Build history of the part. All positions in model axes, mm. Give positions to 0.01 mm unless a question says otherwise; leave off trailing zeros. Write each loop counter-clockwise with the first axis right and the second up, starting at its lowest first coordinate (ties: lowest second). Pieces come first, ordered by that corner, then holes.
from build123d import *

# Parameters (mm, degrees)
F0_W     = 3.9206347639
F0_H     = 6.35
F0_W_2   = 38.6172633823
F0_W_3   = 6.145446312
F1_DEPTH = 3.175
F3_DEPTH = 1.5875
F5_DEPTH = 1.5875


with BuildPart() as f1:
    # F0 (on Front) → F1 (new body, symmetric)
    with BuildSketch(Plane.XZ):
        with BuildLine():
            add(Edge.make_bspline(
                [(-63.5830785449, -61.1632146377), (-60.6032821452, -14.1837314043), (-41.3495043683, 45.8758918628), (10.5261552874, 69.8420151656)],
                knots=[0, 0, 0, 0, 150.514280967, 150.514280967, 150.514280967, 150.514280967], degree=3))
            Line((-63.5830785449, -61.1632146377), (10.5261552874, -61.1632146377))
            Line((10.5261552874, -61.1632146377), (10.5261552874, -54.4388230847))
            Line((10.5261552874, -54.4388230847), (6.6055205235, -54.4388230847))
            Line((6.6055205235, -54.4388230847), (6.6055205235, -48.0888230847))
            Line((6.6055205235, -48.0888230847), (10.5261552874, -48.0888230847))
            Line((10.5261552874, -48.0888230847), (10.5261552874, 69.8420151656))
        make_face()
        with Locations((8.5658379055, -51.2638230847)):
            Rectangle(F0_W, F0_H)
        with Locations((29.8347869785, -51.2638230847)):
            Rectangle(F0_W_2, F0_H)
        with Locations((52.2161418257, -51.2638230847)):
            Rectangle(F0_W_3, F0_H)
    extrude(amount=F1_DEPTH, both=True)

    # F2 (on face) → F3 (join, symmetric)
    with BuildSketch(Plane(origin=(0, 3.175, 0), x_dir=(-1, 0, 0), z_dir=(0, 1, 0))):
        with BuildLine():
            Line((-4.1227932088, 26.3006426394), (-4.1227932088, -61.1632146377))
            Line((-4.1227932088, -61.1632146377), (47.1498034894, -61.1632146377))
            ThreePointArc((47.1498034894, -61.1632146377), (30.1089207689, -12.3925272169), (-4.1227932088, 26.3006426394))
        make_face()
    extrude(amount=F3_DEPTH, both=True)

    # F4 (on face) → F5 (join, symmetric)
    with BuildSketch(Plane.XZ.offset(3.175)):
        with BuildLine():
            Line((-47.3917610943, -61.1632146377), (4.3468987569, -61.1632146377))
            Line((4.3468987569, -61.1632146377), (4.3468987569, 26.0813757777))
            ThreePointArc((4.3468987569, 26.0813757777), (-30.2325786117, -12.3755406522), (-47.3917610943, -61.1632146377))
        make_face()
    extrude(amount=F5_DEPTH, both=True)


solid = f1.part
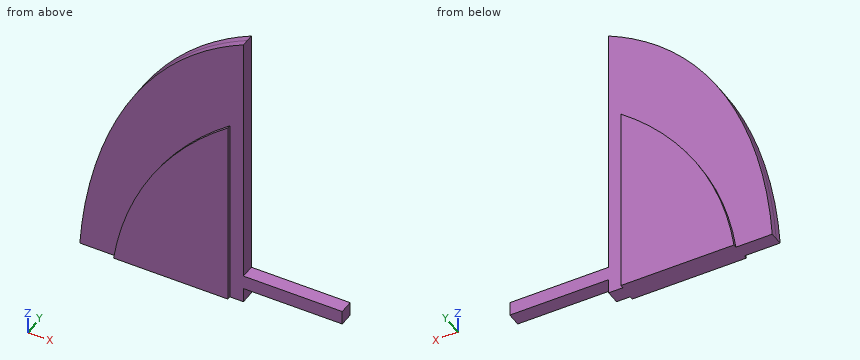
(1) Probe line 1 (Y direction, x = -35.5, z = -4.5) (3 decimals); line 2 (Z direction, x = 41, y = -1.25); line 3 (Z direction, x = -5, y = 2.5). List the from-to ranges inside material, lowest first.
(2) Saw through at A-A, the plane x = 24. List the corners of the cut face in (y, z) (3 decimals), plus the area to 3 significant figures.
(3) Drop flat-ended pins along their axis: pin 1 (1.5 mm diameter, centred on y = 0.5, z = 47, fed in from +X); pin 2 (1.3 mm diameter, centred on y = -4, z = -33, fed in from +X); pin 3 (4 mm diameter, centred on x = 13.5, y = -2.5, fed in from +Z); pin 4 (4 mm diameter, centred on x = -20, z = 4.5, fed in from -Y). Give the stop position or say it passes through.
Computed values:
1. line 1: y = -3.175 to 3.175
1. line 2: z = -54.44 to -48.09
1. line 3: z = -61.16 to 60.99
2. outline: (-3.175, -54.439) - (3.175, -54.439) - (3.175, -48.089) - (-3.175, -48.089) - close
2. area: 40.3 mm2
3. pin 1: stops at x = 10.53
3. pin 2: stops at x = 4.35
3. pin 3: stops at z = -48.09
3. pin 4: stops at y = -4.76
